Geometry: see drawing. Coordinates: mm, zero at the bounding-box minimum. Give positions to 0.01 mm unless a question says otherwise; leave off trailing zeros. Loops run counter-clockwise (first coordinate to the right, second up) from the corner with the lowest first, then second, coordinate; pieces in that order, holes last. Notation, with made-up numbers: (1, 75.25) -> (45, 75.25) arc R21 ccw to (45, 81.25) -> close; hole circle Ø5 at (65, 47.25). An arc over 180 degrees is marked (long way). Return JSON: item names as keys, results as strings. Group by question number.
(1) Draft query along Z for the marked faces 1 and 2. Return one class per face: released by +Z, released by -Z, zero draft, split by the parting line, or undercut.
(2) Cut plane D-D on y = 20. Return loops of the section in (x, z), then the cut area to 3 significant figures.
(3) Cut plane A-A on y = 60. Return loops of the section in (x, z).
(4) Ray query, line 1 (Y direction, x = 20, z = 0.7); line 2 (X direction, y = 19, z = 0.2). Return the intervals inside material, ascending. Write a range as from..to.
(5) Pin query (flat end, axial travel): pin 1 (11.5 mm diameter, centred on x = 20, y = 60, fed in from -Z); pin 2 (7 mm diameter, centred on x = 60, y = 20, fed in from +Z). Return the tip coordinate at first contact, or that it passes through.
(6) Cut plane C-C on z = 0.45. Return loops of the section in (x, y).
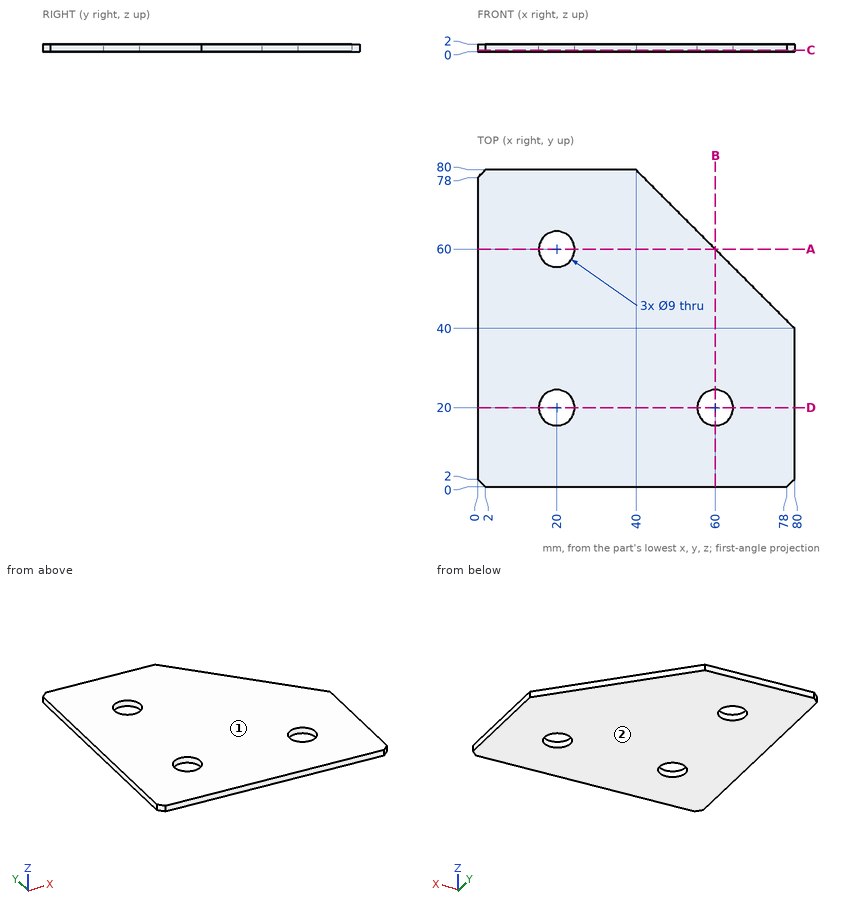
Answers:
{
 "1": {"face 1": "released by +Z", "face 2": "released by -Z"},
 "2": {"outline": "(0, 0) -> (15.5, 0) -> (15.5, 2) -> (0, 2) -> close; (24.5, 0) -> (55.5, 0) -> (55.5, 2) -> (24.5, 2) -> close; (64.5, 0) -> (80, 0) -> (80, 2) -> (64.5, 2) -> close", "area": "124 mm²"},
 "3": {"outline": "(0, 0) -> (15.5, 0) -> (15.5, 2) -> (0, 2) -> close; (24.5, 0) -> (60, 0) -> (60, 2) -> (24.5, 2) -> close"},
 "4": {"line 1": "0..15.5, 24.5..55.5, 64.5..80", "line 2": "0..15.61, 24.39..55.61, 64.39..80"},
 "5": {"pin 1": "z = 0", "pin 2": "through"},
 "6": {"outline": "(0, 2) -> (2, 0) -> (78, 0) -> (80, 2) -> (80, 40) -> (40, 80) -> (2, 80) -> (0, 78) -> close; hole circle Ø9 at (20, 20); hole circle Ø9 at (20, 60); hole circle Ø9 at (60, 20)"}
}
